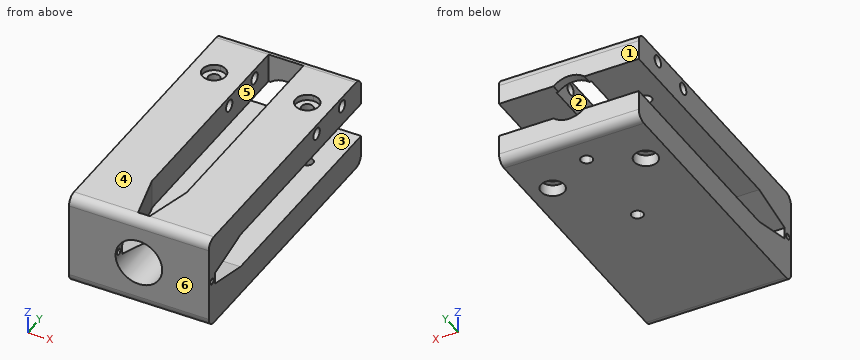
from build123d import *

# Parameters (mm, degrees)
F0_W      = 76.2
F0_H      = 50.8
F0_R      = 12.7
F1_DEPTH  = 152.4
F2_R      = 5.08
F4_DEPTH  = 76.201
F5_W      = 19.05
F5_H      = 116.84
F6_DEPTH  = 19.05
F8_DEPTH  = 50.801
F10_DEPTH = 76.201
F12_DEPTH = 3.175
F13_R     = 3.175
F14_DEPTH = 47.6260001
F15_R     = 3.175
F16_DEPTH = 47.6260001
F17_R     = 6.35
F18_DEPTH = 6.35
F19_R     = 3.175
F20_DEPTH = 76.2010001


with BuildPart() as f1:
    # F0 (on Front) → F1 (new body)
    with BuildSketch(Plane.XZ):
        Rectangle(F0_W, F0_H)
        Circle(F0_R, mode=Mode.SUBTRACT)
    extrude(amount=F1_DEPTH)

    # F2
    f2_edges = [f1.edges().sort_by_distance(p)[0] for p in [
        (0, -152.4, 25.4),
        (0, -152.4, -25.4),
        (0, 0, 25.4),
        (0, 0, -25.4),
    ]]
    fillet(f2_edges, radius=F2_R)

    # F3 (on face) → F4 (cut, through all)
    with BuildSketch(Plane(origin=(-38.1, 0, 0), x_dir=(0, -1, 0), z_dir=(-1, 0, 0))):
        Polygon((12.7, 0), (0, 0), (0, -3.175), (0, -9.525), (120.65, -9.525), (120.65, 0), (88.9, 0), align=None)
        Polygon((0, 3.175), (0, 0), (12.7, 0), (88.9, 0), (120.65, 0), (120.65, 9.525), (0, 9.525), align=None)
        Polygon((120.65, 9.525), (120.65, 0), (139.7, 0), (146.05, 0), (146.05, 3.175), align=None)
        Polygon((139.7, 0), (120.65, 0), (120.65, -9.525), (146.05, -3.175), (146.05, 0), align=None)
    extrude(amount=-F4_DEPTH, mode=Mode.SUBTRACT)

    # F5 (on face) → F6 (cut)
    with BuildSketch(Plane.XY.offset(25.4)):
        Polygon((-3.175, -147.32), (0, -147.32), (3.175, -147.32), (9.525, -121.92), (-9.525, -121.92), align=None)
        with Locations((0, -63.5)):
            Rectangle(F5_W, F5_H)
    extrude(amount=-F6_DEPTH, mode=Mode.SUBTRACT)

    # F7 (on face) → F8 (cut, through all)
    with BuildSketch(Plane(origin=(0, 0, -25.4), x_dir=(1, 0, 0), z_dir=(0, 0, -1))):
        with BuildLine():
            ThreePointArc((0, 20.955), (-3.175, 17.78), (0, 14.605))
            Line((0, 14.605), (0, 17.78))
            Line((0, 17.78), (0, 20.955))
        make_face()
        with BuildLine():
            ThreePointArc((0, 71.755), (-3.175, 68.58), (0, 65.405))
            Line((0, 65.405), (0, 68.58))
            Line((0, 68.58), (0, 71.755))
        make_face()
        with BuildLine():
            Line((0, 68.58), (0, 65.405))
            ThreePointArc((0, 65.405), (2.2450640303, 66.3349359697), (3.175, 68.58))
            ThreePointArc((3.175, 68.58), (2.2450640303, 70.8250640303), (0, 71.755))
            Line((0, 71.755), (0, 68.58))
        make_face()
        with BuildLine():
            Line((0, 17.78), (0, 14.605))
            ThreePointArc((0, 14.605), (2.2450640303, 15.5349359697), (3.175, 17.78))
            ThreePointArc((3.175, 17.78), (2.2450640303, 20.0250640303), (0, 20.955))
            Line((0, 20.955), (0, 17.78))
        make_face()
    extrude(amount=-F8_DEPTH, mode=Mode.SUBTRACT)

    # F9 (on face) → F10 (cut, through all)
    with BuildSketch(Plane(origin=(-38.1, 0, 0), x_dir=(0, -1, 0), z_dir=(-1, 0, 0))):
        with BuildLine():
            ThreePointArc((147.6375, 0), (149.225, -1.5875), (150.8125, 0))
            Line((150.8125, 0), (149.225, 0))
            Line((149.225, 0), (147.6375, 0))
        make_face()
        with BuildLine():
            Line((149.225, 0), (150.8125, 0))
            ThreePointArc((150.8125, 0), (149.225, 1.5875), (147.6375, 0))
            Line((147.6375, 0), (149.225, 0))
        make_face()
    extrude(amount=-F10_DEPTH, mode=Mode.SUBTRACT)

    # F11 (on face) → F12 (cut)
    with BuildSketch(Plane.XY.offset(25.4)):
        with BuildLine():
            ThreePointArc((-19.05, -30.48), (-20.9098719395, -25.9898719395), (-25.4, -24.13))
            ThreePointArc((-25.4, -24.13), (-29.8901280605, -34.9701280605), (-19.05, -30.48))
        make_face()
        with BuildLine():
            ThreePointArc((31.75, -30.48), (29.8901280605, -25.9898719395), (25.4, -24.13))
            ThreePointArc((25.4, -24.13), (20.9098719395, -34.9701280605), (31.75, -30.48))
        make_face()
    extrude(amount=-F12_DEPTH, mode=Mode.SUBTRACT)

    # F13 (on face) → F14 (cut, through all)
    with BuildSketch(Plane.XY.offset(22.225)):
        with Locations((25.4, -30.48)):
            Circle(F13_R)
    extrude(amount=-F14_DEPTH, mode=Mode.SUBTRACT)

    # F15 (on face) → F16 (cut, through all)
    with BuildSketch(Plane.XY.offset(22.225)):
        with Locations((-25.4, -30.48)):
            Circle(F15_R)
    extrude(amount=-F16_DEPTH, mode=Mode.SUBTRACT)

    # F17 (on face) → F18 (cut)
    with BuildSketch(Plane(origin=(0, 0, -25.4), x_dir=(1, 0, 0), z_dir=(0, 0, -1))):
        with Locations((-25.4, 30.48)):
            Circle(F17_R)
        with Locations((25.4, 30.48)):
            Circle(F17_R)
    extrude(amount=-F18_DEPTH, mode=Mode.SUBTRACT)

    # F19 (on face) → F20 (cut, through all)
    with BuildSketch(Plane(origin=(-38.1, 0, 0), x_dir=(0, -1, 0), z_dir=(-1, 0, 0))):
        with BuildLine():
            ThreePointArc((47.625, 20.32), (44.45, 23.495), (41.275, 20.32))
            ThreePointArc((41.275, 20.32), (44.45, 17.145), (47.625, 20.32))
        make_face()
        with Locations((19.05, 20.32)):
            Circle(F19_R)
    extrude(amount=-F20_DEPTH, mode=Mode.SUBTRACT)


solid = f1.part
Read the model definition and answer for the solid it produces. Units are mm, in the model's axes. Face numbers are marked on the shaded views. A direction names the side the tool comes from. Give positions to 0.01 mm unless a question says otherwise; leave off trailing zeros. Write each loop counter-clockwise with the first axis right and the second up, starting at its lowest first coordinate (ties: lowest second). Pieces come first, ordered by that corner, then holes. Notation, with made-up numbers: (43.5, 70.25) - (55.5, 70.25) arc R27 cw to (55.5, 99.25) - close; hole circle Ø5 at (30.25, 5). An arc over 180 degrees is marked (long way). Answer in a Markdown table with one row per item. Add a question column.
Item 1: Find the intervals of material crossed by L1, parallel to X at y = -30.48, z = 24.4 (3 decimals); L2, parallel to X at y = -30.48, z = -23.25; L3, parallel to X at y = -95, z = 20 (3 decimals), in increasing order.
Item 2: Determine the mould class of the marked faces 4, 5 and 6 for opening direction Y: pulls with the +Y half, pulls with the -Y half, needs draft (parallel to the pull), parting line crosses it, or undercut.
Item 3: Section D-D, the plane y = -113.5 is taken. Write down the section's boundary in (x, z) (3 decimals).
Item 4: Flat-ended cylindrical pins translate along their axes: P1, Ø8, axis at x = -1.5, y = -72.5, coming from the +Z side; P2, Ø5, axis at x = -20.5, z = 0, coming from the +Y side; P3, Ø11.5, axis at x = 25.4, y = -30.48, coming from the -Z side. Find the tip coordinate at first contact, or state that the pin passes through.
Item 5: A tool of negligible diameter and unlimited length cuts with its end or side. For the marked faces 1, 2 and 3, from which of +Z, -Z, +X, -X, +Y, -Y can it reach the whole face along a straight path? Write none if from no direction.
Item 6: Section A-A, the plane y = -44.45 is taken. Write down the section's boundary in (x, z) (3 decimals), and give its area (3 significant figures).
Item 7: Section B-B, the plane x = -15.5 is taken. Count the separate pieces of the cut face and the enclosed holes in it, and give its area (3 significant figures).
Recorded:
| question | item | result |
|---|---|---|
| 1 | L1 | x = -38.1 to -31.75, -19.05 to -9.525, 9.525 to 19.05, 31.75 to 38.1 |
| 1 | L2 | x = -38.1 to -31.75, -19.05 to 19.05, 31.75 to 38.1 |
| 1 | L3 | x = -38.1 to -9.525, 9.525 to 38.1 |
| 2 | face 4 | needs draft |
| 2 | face 5 | undercut |
| 2 | face 6 | pulls with the -Y half |
| 3 | outline | (-38.1, -25.4) - (38.1, -25.4) - (38.1, -9.525) - (8.4, -9.525) arc R12.7 cw to (-8.4, -9.525) - (-38.1, -9.525) - close; (-38.1, 9.525) - (-9.525, 9.525) - (-9.525, 25.4) - (-38.1, 25.4) - close; (9.525, 9.525) - (38.1, 9.525) - (38.1, 25.4) - (9.525, 25.4) - close |
| 4 | P1 | stops at z = -11.45 |
| 4 | P2 | stops at y = -146.05 |
| 4 | P3 | stops at z = -19.05 |
| 5 | face 1 | +Z, -Z, +X, -X, +Y |
| 5 | face 2 | +Z |
| 5 | face 3 | +X, -X, +Y |
| 6 | outline | (-38.1, -25.4) - (38.1, -25.4) - (38.1, -9.525) - (8.4, -9.525) arc R12.7 cw to (-8.4, -9.525) - (-38.1, -9.525) - close; (-38.1, 9.525) - (-9.525, 9.525) - (-9.525, 17.145) - (-38.1, 17.145) - close; (-38.1, 23.495) - (-9.525, 23.495) - (-9.525, 25.4) - (-38.1, 25.4) - close; (9.525, 9.525) - (38.1, 9.525) - (38.1, 17.145) - (9.525, 17.145) - close; (9.525, 23.495) - (38.1, 23.495) - (38.1, 25.4) - (9.525, 25.4) - close |
| 6 | area | 1,720 mm2 |
| 7 | separate pieces | 1 |
| 7 | enclosed holes | 3 |
| 7 | area | 5,030 mm2 |
